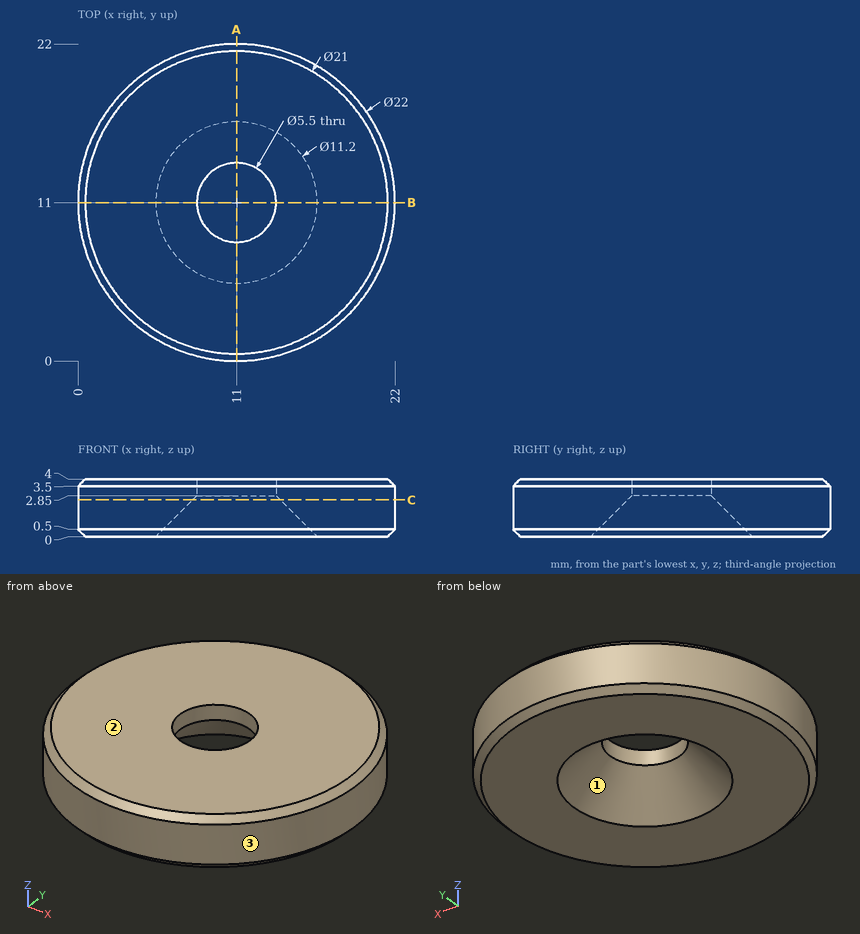
Could you check a few things on this drawing? It's one solid part, dimensions in mm from its lowest x, y, z. Give positions to 0.01 mm unless a question says otherwise; leave off trailing zeros. Write each loop counter-clockwise with the first axis right and the second up, starting at its lowest first coordinate (ties: lowest second). Pieces come first, ordered by that corner, then holes. Notation, with made-up numbers: (73.25, -3.75) -> (85.25, -3.75) arc R24 ccw to (85.25, 31.25) -> close; hole circle Ø3 at (49, -32). An arc over 180 degrees is marked (long way). Write each question's results on one line, items separated by ' | '.
1. Will these pins go through, and if not, where does the flat tip stop? pin 1 Ø7 at (x, y) = (11, 11) entering from +Z; pin 2 Ø1 at (y, z) = (14, 1) entering from -X.
Check sheet entries:
pin 1: stops at z = 4 | pin 2: stops at x = 0.29
2. I want a section at A-A, the plane x = 11. Write out the boundary of the cut face in (y, z), then the cut area to 3 significant figures.
Check sheet entries:
outline: (0, 0.5) -> (0.5, 0) -> (5.4, 0) -> (8.25, 2.85) -> (8.25, 4) -> (0.5, 4) -> (0, 3.5) -> close; (13.75, 2.85) -> (16.6, 0) -> (21.5, 0) -> (22, 0.5) -> (22, 3.5) -> (21.5, 4) -> (13.75, 4) -> close | area: 57.4 mm²
3. I need wall thicknesses on L1, parallel to Y at x = 11, z = 3.15; L2, parallel to X at y = 10.25, z = 0.45; L3, parallel to X at y = 10.25, z = 1. Which ranges of each line are inside material? Lowest first, please.
Check sheet entries:
L1: y = 0 to 8.25, 13.75 to 22 | L2: x = 0.08 to 5.9, 16.1 to 21.92 | L3: x = 0.03 to 6.46, 15.54 to 21.97
4. If we mould it in two halves opening along X, with no side actions, what happens to the marked faces 1, 2 and 3? For each: released by +X, released by -X, zero draft, split by the parting line, or undercut.
Check sheet entries:
face 1: undercut | face 2: zero draft | face 3: split by the parting line
5. I want a section at C-C, the plane z = 2.55. Write out the boundary of the cut face in (x, y), then the cut area to 3 significant figures.
Check sheet entries:
outline: circle Ø22 at (11, 11); hole circle Ø6.1 at (11, 11) | area: 351 mm²
